Verification items for the finished model (mm, model axes). A direction names the side the tool comes from. Give positions to 0.01 mm unless a question says otherwise; leave off trailing zeros. Loops run counter-clockwise (first coordinate to the right, second up) from the corner with the lowest first, then second, coordinate; pieces in that order, holes last. Notation, with made-up numbers: (33, 81) -> (51, 81) arc R23 ccw to (51, 91) -> close; hole circle Ø9 at (33, 15). An arc over 180 degrees is marked (long way). Answer in a Markdown table with one row per item. Add a question column.
Q1. Section check B-B on y = 10. Enter the section's corners in (x, z).
Q2. Section check A-A on z = -45. Enter the section's corners in (x, y), and give its area (3 significant figures).
Q3. Section check C-C on y = 3. Enter the section's corners in (x, z).
Q4. Material ranges on probe 1 along X at (y, z) = (17, -45.5), recorded low to high.
Q5. Section check D-D on z = -12. Enter the section's corners in (x, y).
Q6. Set-up check for faces 1 (the face through (-46.97, 10.96, -42.69)), 2 (the face through (-49, 10, -45)): record each of +Z, -Z, +X, -X, +Y, -Y from which the full face is reachable in a straight line by a thin tool's end or side.
Autodesk Inventor part; units mm, degrees
ref_plane "YZ Plane" through (0, 0, 0) normal (1, 0, 0) x (0, 1, 0)
ref_plane "XZ Plane" through (0, 0, 0) normal (0, 1, 0) x (-1, 0, 0)
ref_plane "XY Plane" through (0, 0, 0) normal (0, 0, 1) x (1, 0, 0)
sketch "Sketch1" plane through (0, 0, 0) normal (0, 1, 0) x (-1, 0, 0)
  line L0 (0, 0) -> (45, 0)
  line L1 (45, 0) -> (45, -55)
  line L2 (45, -55) -> (0, -55)
  line L3 (0, -55) -> (0, 0)
  dimension "d0" = 45
  dimension "d1" = 55
extrude "Extrusion1" add sketch "Sketch1" along normal blind 20
sketch "Sketch2" plane through (-45, 0, -55) normal (-1, 0, 0) x (0, 0, 1)
  circle A0 centre (10, 10) radius 2.5
  line L0 (0, 0) -> (0, 20)
  line L1 (0, 0) -> (55, 0)
  dimension "d4" = 10
  dimension "d5" = 10
  dimension "d6" = 5
extrude "Extrusion2" add sketch "Sketch2" along normal blind 4
properties part number "servo mg958 dummy"
Taken from the geometry:
| question | item | result |
|---|---|---|
| 1 | outline | (-49, -47.5) -> (-45, -47.5) -> (-45, -55) -> (0, -55) -> (0, 0) -> (-45, 0) -> (-45, -42.5) -> (-49, -42.5) -> close |
| 2 | outline | (-49, 7.5) -> (-45, 7.5) -> (-45, 0) -> (0, 0) -> (0, 20) -> (-45, 20) -> (-45, 12.5) -> (-49, 12.5) -> close |
| 2 | area | 920 mm² |
| 3 | outline | (-45, -55) -> (0, -55) -> (0, 0) -> (-45, 0) -> close |
| 4 | probe 1 | x = -45 to 0 |
| 5 | outline | (-45, 0) -> (0, 0) -> (0, 20) -> (-45, 20) -> close |
| 6 | face 1 | -X |
| 6 | face 2 | +Z, -Z, -X, +Y, -Y |
